Verification items for the finished model (mm, model axes). A direction names the side the tool comes from. Round coordinates to 2 decimals unless told otherwise and drop trailing zeros. One line per question, with ' | ' between items. Start each with the question number.
Q1. Tool access check on faces 1 (the face through (-1, -10, 5)), 2 (the face through (71.451, -6.335, 5.421)), 3 (the face through (-71.451, 6.335, 5.421)). Record the directions out of +Z, -Z, +X, -X, +Y, -Y that give a thin tool (end or side, any length) a straight path to the whole face; none if there is none.
Q2. Thickness scan on line 1 along Y through (x, z) = (-72, 5); line 2 along Z through (x, y) = (72, 5). Record the ranges inside material, lowest first. Write a range as from..to.
Q3. Release check for a two-part mould opening along Z. For faces 4 (the face through (-75, 0, 5)), 5 (the face through (-1, 0, 10)), 6 (the face through (71.451, 3.665, 5.421)), 7 (the face through (-71.451, -3.665, 5.421)) record: released by +Z, released by -Z, zero draft, split by the parting line, or undercut.
Q4. Gauge pin test, flat ends, axial feed: pin 1 (3 mm diameter, centred on y = -5, z = 5, fed in from -X); pin 2 (2.5 mm diameter, centred on y = 5, z = 5, fed in from -X); pin 3 (1.7 mm diameter, centred on y = 5, z = 5, fed in from +X). Record the tip position at first contact, or that the pin passes through.
from build123d import *

# Parameters (mm, degrees)
F0_W     = 150
F0_H     = 20
F1_DEPTH = 10
F3_D     = 2.8
F3_DEPTH = 7
F3_TIP   = 0.8412048666
F5_D     = 2.8
F5_DEPTH = 7
F5_TIP   = 0.8412048666


with BuildPart() as f1:
    # F0 (on Top) → F1 (new body)
    with BuildSketch(Plane.XY):
        Rectangle(F0_W, F0_H)
    extrude(amount=F1_DEPTH)

    # F3
    with Locations(Plane(origin=(-75, 0, 0), x_dir=(0, -1, 0), z_dir=(-1, 0, 0))):
        with Locations((-5, 5), (5, 5)):
            Hole(F3_D / 2, depth=F3_DEPTH)
            with Locations((0, 0, -(F3_DEPTH + F3_TIP / 2))):  # 118° drill point
                Cone(0, F3_D / 2, F3_TIP, mode=Mode.SUBTRACT)

    # F5
    with Locations(Plane.YZ.offset(75)):
        with Locations((-5, 5), (5, 5)):
            Hole(F5_D / 2, depth=F5_DEPTH)
            with Locations((0, 0, -(F5_DEPTH + F5_TIP / 2))):  # 118° drill point
                Cone(0, F5_D / 2, F5_TIP, mode=Mode.SUBTRACT)


solid = f1.part
Determined:
1) face 1: +Z, -Z, +X, -X, -Y | face 2: +X | face 3: -X
2) line 1: y = -10..-6.4, -3.6..3.6, 6.4..10 | line 2: z = 0..3.6, 6.4..10
3) face 4: zero draft | face 5: released by +Z | face 6: undercut | face 7: undercut
4) pin 1: stops at x = -75 | pin 2: stops at x = -67.91 | pin 3: stops at x = 67.67
